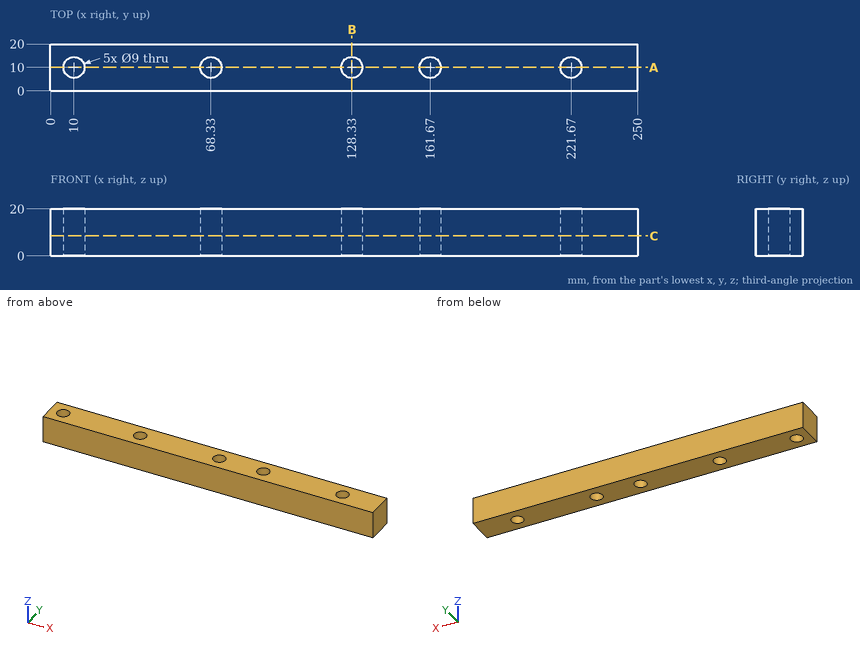
For this review, use the dimensioned drawing (mm, ordinates from the lowest corner) and the shaded views. Coordinates: 2 decimals unless noted, no trailing zeros. Loops run counter-clockwise (first coordinate to the right, second up) from the corner with the lowest first, then second, coordinate; pieces in that order, holes last. Notation, with made-up numbers: (57, 79.5) -> (113, 79.5) arc R7 cw to (113, 85.5) -> close; hole circle Ø7 at (88.25, 9.5). An arc over 180 degrees is marked (long way). Use a Markdown table: item, result. Add a question column.
Item 1: We need section B-B, the plane x = 128.33. Write out the cut boundary in (y, z), and give its area (3 significant figures).
Item 2: Wall thickness on L1, parallel to X at y = 8.25, z = 12; L2, parallel to Y at x = 10, z = 10.5; L3, parallel to X at y = 9, z = 14.25: over which ranges is each line inside the solid? List them lowest first. Write a range as from..to.
Item 3: Clearance check with a flat-ended pin moving along its axis: P1, Ø12, axis at x = 153, z = 10.5, coming from the -Y side. State where the tip first meets the part, or that it passes through.
Item 4: We need section A-A, the plane y = 10. Write out the cut boundary in (x, z), and give its area (3 significant figures).
Item 5: We need section C-C, the plane z = 8.5. Write out the cut boundary in (x, y).
Numbers:
| question | item | result |
|---|---|---|
| 1 | outline | (0, 0) -> (5.5, 0) -> (5.5, 20) -> (0, 20) -> close; (14.5, 0) -> (20, 0) -> (20, 20) -> (14.5, 20) -> close |
| 1 | area | 220 mm^2 |
| 2 | L1 | x = 0..5.85, 14.15..64.18, 72.48..124.18, 132.48..157.52, 165.82..217.52, 225.82..250 |
| 2 | L2 | y = 0..5.5, 14.5..20 |
| 2 | L3 | x = 0..5.61, 14.39..63.94, 72.72..123.94, 132.72..157.28, 166.06..217.28, 226.06..250 |
| 3 | P1 | stops at y = 0 |
| 4 | outline | (0, 0) -> (5.5, 0) -> (5.5, 20) -> (0, 20) -> close; (14.5, 0) -> (63.83, 0) -> (63.83, 20) -> (14.5, 20) -> close; (72.83, 0) -> (123.83, 0) -> (123.83, 20) -> (72.83, 20) -> close; (132.83, 0) -> (157.17, 0) -> (157.17, 20) -> (132.83, 20) -> close; (166.17, 0) -> (217.17, 0) -> (217.17, 20) -> (166.17, 20) -> close; (226.17, 0) -> (250, 0) -> (250, 20) -> (226.17, 20) -> close |
| 4 | area | 4,100 mm^2 |
| 5 | outline | (0, 0) -> (250, 0) -> (250, 20) -> (0, 20) -> close; hole circle Ø9 at (10, 10); hole circle Ø9 at (68.33, 10); hole circle Ø9 at (128.33, 10); hole circle Ø9 at (161.67, 10); hole circle Ø9 at (221.67, 10) |
